For this review, use the dimensioned drawing (mm, ordinates from the lowest corner) and the shaded views. Give positions to 0.01 mm unless a question says otherwise; leave off trailing zeros. Loops run counter-clockwise (first coordinate to the right, second up) from the corner with the lowest first, then second, coordinate; pieces in that order, holes last. Notation, with made-up numbers: (25.5, -1.5) -> (61.5, -1.5) arc R10 cw to (61.5, 2.5) -> close; hole circle Ø1 at (-27, 77.25). An arc over 180 degrees is marked (long way). Write each question's results on one line, items separated by ' | '. Start each with the question number.
Q1. We need section B-B (x = 83.45). Write out the cut boundary in (y, z), plus the area to 3 significant figures.
Q2. We need section C-C (z = 10.5). Write out the cut boundary in (x, y).
Q3. We need section A-A (x = 69). Write out the cut boundary in (y, z).
Q4. We need section D-D (y = 24). Write out the cut boundary in (x, z).
Q5. Wall thickness on L1, parallel to X at y = 1, z = 69; L2, parallel to X at y = 27, z = 69: over which ranges is each line inside the solid? List them lowest first. Write a range as [from, to].
Q6. Insertion check: pin 1 Ø4 at (x, y) = (119, 61) entering from +Z; pin 2 Ø1.5 at (y, z) = (65.5, 94) entering from +X; pin 3 Ø2 at (x, y) = (61.5, 51.5) entering from -Z; pin 4 Ø6 at (x, z) = (69, 69) entering from -Y. Each pin has a flat end and moves straight along its axis. Give the tip position at first contact, or say it passes through.
Q7. Mouldability with a two-part tool opening along Z and no side actions: class the marked faces 1, 2 and 3 as released by +Z, released by -Z, zero draft, split by the parting line, or undercut.
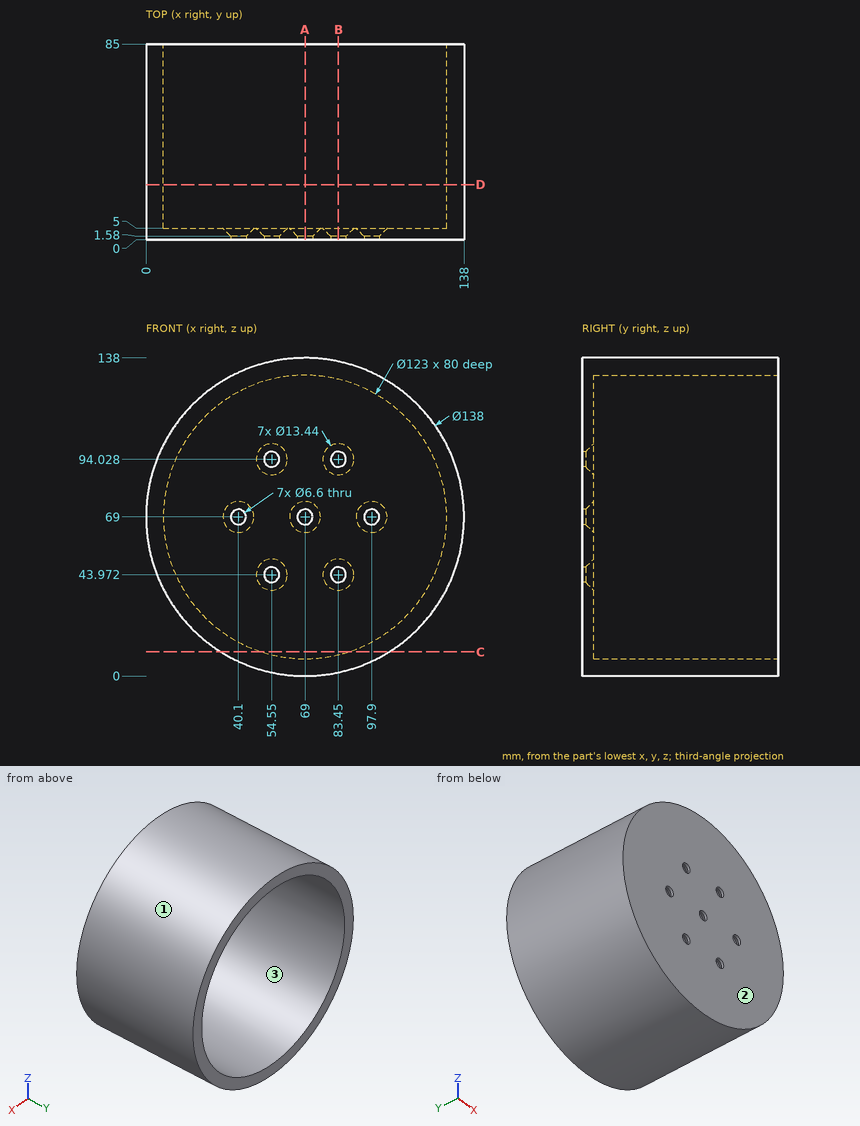
Output:
1) outline: (0, 1.53) -> (85, 1.53) -> (85, 9.22) -> (5, 9.22) -> (5, 37.25) -> (1.58, 40.67) -> (0, 40.67) -> close; (0, 47.27) -> (1.58, 47.27) -> (5, 50.69) -> (5, 87.31) -> (1.58, 90.73) -> (0, 90.73) -> close; (0, 97.33) -> (1.58, 97.33) -> (5, 100.75) -> (5, 128.78) -> (85, 128.78) -> (85, 136.47) -> (0, 136.47) -> close | area: 1,820 mm2
2) outline: (32.41, 0) -> (105.59, 0) -> (105.59, 85) -> (87.97, 85) -> (87.97, 5) -> (50.03, 5) -> (50.03, 85) -> (32.41, 85) -> close
3) outline: (0, 0) -> (85, 0) -> (85, 7.5) -> (5, 7.5) -> (5, 62.28) -> (1.58, 65.7) -> (0, 65.7) -> close; (0, 72.3) -> (1.58, 72.3) -> (5, 75.72) -> (5, 130.5) -> (85, 130.5) -> (85, 138) -> (0, 138) -> close
4) outline: circle Ø138 at (69, 69); hole circle Ø123 at (69, 69)
5) L1: [0, 36.8], [43.4, 65.7], [72.3, 94.6], [101.2, 138] | L2: [0, 7.5], [130.5, 138]
6) pin 1: z = 118.57 | pin 2: x = 133.6 | pin 3: z = 0.31 | pin 4: through
7) face 1: split by the parting line | face 2: zero draft | face 3: undercut
